Geometry check sheet. Reference: the model listing, model coordinates, mm. A direction names the side the tool comes from. Round coordinates to 2 decimals unless told otherwise and drop trailing zeros. Order: outer loops, then holes, each group sorted by start corner. A loop starts at its lowest first (then second) coordinate and runs counter-clockwise, first axis right, second up. Notation, with made-up numbers: (48.25, 57) - (63.25, 57) arc R11 cw to (63.25, 77) - close; hole circle Ø7 at (-10, 47). An arc over 180 degrees is marked (long way). Use a Markdown table: item, result. Add a question column.
(1) Thickness scan on line 1 along Y through (x, z) = (54.35, 16.4); line 2 along X through (y, z) = (85.35, 12.1); line 3 along Z through (x, y) = (19.05, 46). Record the ranges inside material, lowest first. Write a range as [from, to].
(2) Section check A-A on x = 19.05. Record the boundary of the cut face in (y, z), then the cut area to 3 significant figures.
(3) Mould release check, pull along Z, two halves, no side actions. Record for faces 5 (the face through (56, 53, 13.335)), 6 (the face through (69, 0, 10)), 7 (the face through (13, 69, 10)): released by +Z, released by -Z, zero draft, split by the parting line, or undercut.
(4) Access from +Z, -Z, +X, -X, +Y, -Y to the whole of each face (thin tool, end or side, straight path). Record for faces 1 (the face through (18.977, 26.926, 2.544)), 2 (the face through (69, 3, 2.032)), 3 (the face through (81.182, 54.897, 16.152)), 4 (the face through (70, 83, 9.525)).
(5) Gauge pin test, flat ends, axial feed: P1, Ø9, axis at x = 54, y = 84, coming from the +Z side; P2, Ø2.5, axis at x = 83.5, y = 55.5, coming from the +Z side (3 decimals); P3, Ø3, axis at x = 66.5, z = 5, coming from the +Y side; P4, Ø6, axis at x = 115.5, z = 8, coming from the +Y side. Record the tip position at first contact, or that the pin passes through.
(6) Section check D-D on x = 54.35. Record the boundary of the cut face in (y, z) (3 decimals).
(7) Section check B-B on y = 54.35. Record the boundary of the cut face in (x, z) (3 decimals).
(8) Section check C-C on x = 75. Record the boundary of the cut face in (y, z) (3 decimals), then the cut area to 3 significant figures.
Autodesk Inventor part; units mm, degrees
ref_plane "YZ Plane" through (0, 0, 0) normal (1, 0, 0) x (0, 1, 0)
ref_plane "XZ Plane" through (0, 0, 0) normal (0, 1, 0) x (-1, 0, 0)
ref_plane "XY Plane" through (0, 0, 0) normal (0, 0, 1) x (1, 0, 0)
sketch "Sketch1" plane through (0, 0, 0) normal (0, 0, 1) x (1, 0, 0)
  line L0 (0, 0) -> (139.7, 0)
  line L1 (139.7, 0) -> (139.7, 82.55)
  line L2 (139.7, 82.55) -> (0, 82.55)
  line L3 (0, 82.55) -> (0, 0)
  line L4 (95.25, 82.55) -> (44.45, 82.55)
  line L5 (44.45, 82.55) -> (44.45, 95.25)
  line L6 (44.45, 95.25) -> (95.25, 95.25)
  line L7 (95.25, 95.25) -> (95.25, 82.55)
  point P0 (69.85, 82.55)
  dimension "d0" = 139.7
  dimension "d1" = 82.55
  dimension "d2" = 12.7
  dimension "d3" = 50.8
  dimension "d4" = 25.4
  dimension "d62" = 69.85
extrude "Extrusion1" add sketch "Sketch1" along normal blind 19.05
sketch "Sketch2" plane through (0, 0, 0) normal (0, 0, -1) x (-1, 0, 0)
  line L0 (-44.45, 82.55) -> (0, 82.55)
  line L1 (-139.7, 0) -> (-139.7, 82.55)
  point P0 (0, 0)
  point P1 (-69.85, 69.85)
  dimension "d7" = 12.7
  dimension "d8" = 69.85
hole "Hole1" at (69.85, 69.85, 0) direction (0, 0, 1) diameter 22 depth 25.4 tip angle 118
sketch "Sketch3" plane through (0, 0, 0) normal (0, 0, -1) x (-1, 0, 0)
  line L0 (-91.44, 48.26) -> (-48.26, 48.26)
  line L1 (-48.26, 48.26) -> (-48.26, 91.44)
  line L2 (-48.26, 91.44) -> (-91.44, 91.44)
  line L3 (-91.44, 91.44) -> (-91.44, 48.26)
  line L4 (-91.44, 48.26) -> (-48.26, 91.44) construction
  line L5 (-48.26, 48.26) -> (-91.44, 91.44) construction
  line L6 (-44.45, 82.55) -> (0, 82.55)
  line L7 (-95.25, 95.25) -> (-44.45, 95.25)
  line L8 (-91.44, 91.44) -> (-48.26, 91.44)
  line L9 (-48.26, 91.44) -> (-48.26, 95.25)
  line L10 (-48.26, 95.25) -> (-91.44, 95.25)
  line L11 (-91.44, 95.25) -> (-91.44, 91.44)
  line L12 (-139.7, 0) -> (-139.7, 82.55)
  point P0 (0, 0)
  point P1 (-69.85, 69.85)
  dimension "d16" = 12.7
  dimension "d17" = 43.18
  dimension "d18" = 43.18
  dimension "d21" = 69.85
  dimension "d22" = 43.18
extrude "Extrusion2" cut sketch "Sketch3" against normal blind 9.525
sketch "Sketch4" plane through (0, 0, 19.05) normal (0, 0, 1) x (1, 0, 0)
  line L0 (54.35, 54.35) -> (85.35, 54.35)
  line L1 (85.35, 54.35) -> (85.35, 85.35)
  line L2 (85.35, 85.35) -> (54.35, 85.35)
  line L3 (54.35, 85.35) -> (54.35, 54.35)
  line L4 (54.35, 54.35) -> (85.35, 85.35) construction
  line L5 (85.35, 54.35) -> (54.35, 85.35) construction
  line L6 (139.7, 82.55) -> (95.25, 82.55)
  line L7 (139.7, 0) -> (139.7, 82.55)
  point P0 (0, 0)
  point P1 (69.85, 69.85)
  dimension "d23" = 12.7
  dimension "d24" = 69.85
  dimension "d25" = 31
  dimension "d26" = 31
hole "Hole2" at (54.35, 85.35, 19.05) at (54.35, 54.35, 19.05) at (85.35, 85.35, 19.05) at (85.35, 54.35, 19.05) direction (0, 0, -1) diameter 3.4036 end through all counterbore diameter 8.4074 counterbore depth 5.715
sketch "Sketch5" plane through (0, 0, 0) normal (0, -1, 0) x (1, 0, 0)
  line L0 (120.65, 9.525) -> (19.05, 9.525)
  line L1 (0, 0) -> (139.7, 0)
  line L2 (139.7, 0) -> (139.7, 19.05)
  dimension "d34" = 101.6
  dimension "d35" = 9.525
  dimension "d36" = 19.05
hole "Hole3" at (120.65, 0, 9.525) at (19.05, 0, 9.525) direction (0, 1, 0) diameter 9.6012 end through all
sketch "Sketch6" plane through (0, 0, 0) normal (0, 0, -1) x (-1, 0, 0)
  line L0 (-120.65, 28.575) -> (-19.05, 28.575)
  line L1 (-44.45, 82.55) -> (0, 82.55)
  line L2 (0, 82.55) -> (0, 0)
  dimension "d44" = 101.6
  dimension "d45" = 53.975
  dimension "d46" = 19.05
hole "Hole4" at (120.65, 28.575, 0) at (19.05, 28.575, 0) direction (0, 0, 1) diameter 3.302 depth 12.2936 tip angle 118
sketch "Sketch7" plane through (0, 0, 0) normal (-1, 0, 0) x (0, 0, 1)
  line L0 (9.525, 95.25) -> (9.525, 48.26)
  line L1 (9.525, 69.055) -> (9.525, 11.905)
  point P0 (0, 0)
  point P1 (9.525, 89.85)
  dimension "d54" = 57.15
hole "Hole5" at (0, 69.055, 9.525) at (0, 11.905, 9.525) direction (1, 0, 0) diameter 3.302 depth 12.2936 tip angle 118
sketch "Sketch8" plane through (139.7, 0, 0) normal (1, 0, 0) x (0, 0, -1)
  line L0 (-19.05, 82.55) -> (-19.05, 0)
  line L1 (0, 0) -> (-19.05, 0)
  point P0 (-9.525, 12.7)
  point P1 (-9.525, 69.85)
  dimension "d87" = 57.15
  dimension "d88" = 9.525
  dimension "d89" = 9.525
  dimension "d90" = 12.7
sketch "Sketch9" plane through (0, 0, 0) normal (0, 0, -1) x (-1, 0, 0)
  line L0 (-139.7, 41.275) -> (0, 41.275)
  line L1 (0, 0) -> (-139.7, 0)
  line L2 (-101.6, 31.369) -> (-38.1, 31.369)
  line L3 (0, 82.55) -> (0, 0)
  line L4 (-44.45, 82.55) -> (0, 82.55)
  line L5 (0, 82.55) -> (-31.75, 41.275)
  line L6 (-17.1517, 76.4998) -> (-38.7838, 52.9606)
  point P0 (-27.3538, 68.7266)
  dimension "d63" = 41.275
  dimension "d64" = 9.906
  dimension "d65" = 139.7
  dimension "d66" = 0
  dimension "d67" = 31.75
  dimension "d68" = 9.906
  dimension "d69" = 12.7
  dimension "d71" = 63.5
  dimension "d72" = 38.1
  dimension "d101" = 11.43
hole "Hole6" at (27.3538, 68.7266, 0) at (38.1, 31.369, 0) at (101.6, 31.369, 0) direction (0, 0, 1) diameter 3.302 depth 12.2936 tip angle 118
hole "Hole8" at (139.7, 12.7, 9.525) at (139.7, 69.85, 9.525) direction (-1, 0, 0) diameter 3.302 depth 12.2936 tip angle 118
sketch "Sketch10" plane through (0, 0, 0) normal (0, -1, 0) x (1, 0, 0)
  point P0 (0, 0)
sketch "Sketch11" plane through (0, 0, 0) normal (0, -1, 0) x (1, 0, 0)
  line L0 (139.7, 0) -> (95.25, 0)
  line L1 (0, 0) -> (0, 19.05)
  line L2 (139.7, 0) -> (0, 0)
  line L3 (0, 0) -> (0, 2.032)
  line L4 (0, 2.032) -> (139.7, 2.032)
  line L5 (139.7, 2.032) -> (139.7, 0)
  dimension "d98" = 2.032
extrude "Extrusion3" cut sketch "Sketch11" against normal blind 6.35
properties part number "back mount"
Check sheet entries:
| question | item | result |
|---|---|---|
| 1 | line 1 | y = [0, 50.15], [58.55, 81.15], [89.55, 95.25] |
| 1 | line 2 | x = [44.45, 52.65], [56.05, 83.65], [87.05, 95.25] |
| 1 | line 3 | z = [0, 4.72], [14.33, 19.05] |
| 2 | outline | (0, 2.03) - (6.35, 2.03) - (6.35, 0) - (26.92, 0) - (26.92, 4.72) - (0, 4.72) - close; (0, 14.33) - (82.55, 14.33) - (82.55, 19.05) - (0, 19.05) - close; (30.23, 0) - (82.55, 0) - (82.55, 4.72) - (30.23, 4.72) - close |
| 2 | area | 751 mm2 |
| 3 | face 5 | released by +Z |
| 3 | face 6 | zero draft |
| 3 | face 7 | undercut |
| 4 | face 1 | -Z |
| 4 | face 2 | -Z, +X, -X, -Y |
| 4 | face 3 | +Z |
| 4 | face 4 | -Z, +Y |
| 5 | P1 | stops at z = 19.05 |
| 5 | P2 | stops at z = 13.335 |
| 5 | P3 | stops at y = 48.26 |
| 5 | P4 | stops at y = 82.55 |
| 6 | outline | (0, 2.032) - (6.35, 2.032) - (6.35, 0) - (48.26, 0) - (48.26, 9.525) - (52.648, 9.525) - (52.648, 13.335) - (50.146, 13.335) - (50.146, 19.05) - (0, 19.05) - close; (56.052, 9.525) - (83.648, 9.525) - (83.648, 13.335) - (81.146, 13.335) - (81.146, 19.05) - (58.554, 19.05) - (58.554, 13.335) - (56.052, 13.335) - close; (87.052, 9.525) - (95.25, 9.525) - (95.25, 19.05) - (89.554, 19.05) - (89.554, 13.335) - (87.052, 13.335) - close |
| 7 | outline | (0, 0) - (48.26, 0) - (48.26, 9.525) - (52.648, 9.525) - (52.648, 13.335) - (50.146, 13.335) - (50.146, 19.05) - (0, 19.05) - close; (56.052, 9.525) - (83.648, 9.525) - (83.648, 13.335) - (81.146, 13.335) - (81.146, 19.05) - (58.554, 19.05) - (58.554, 13.335) - (56.052, 13.335) - close; (87.052, 9.525) - (91.44, 9.525) - (91.44, 0) - (139.7, 0) - (139.7, 19.05) - (89.554, 19.05) - (89.554, 13.335) - (87.052, 13.335) - close; hole circle Ø9.601 at (19.05, 9.525); hole circle Ø9.601 at (120.65, 9.525) |
| 8 | outline | (0, 2.032) - (6.35, 2.032) - (6.35, 0) - (48.26, 0) - (48.26, 9.525) - (60.13, 9.525) - (60.13, 19.05) - (0, 19.05) - close; (79.57, 9.525) - (95.25, 9.525) - (95.25, 19.05) - (79.57, 19.05) - close |
| 8 | area | 1,170 mm2 |
